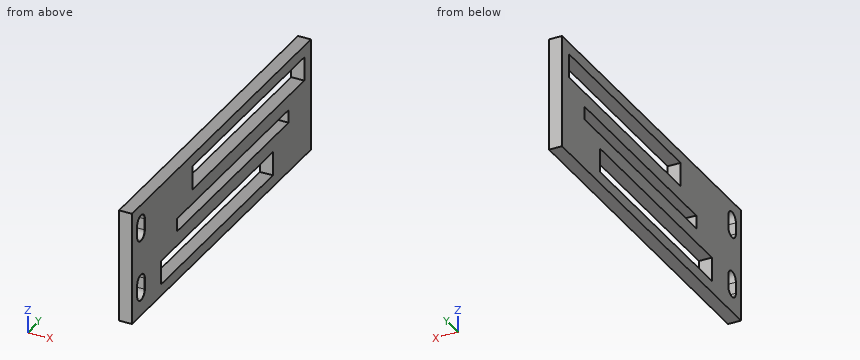
```python
from build123d import *

# Parameters (mm, degrees)
SKETCH1_W                = 26
SKETCH1_H                = 80
BOSS_EXTRUDE1_DEPTH      = 3
SKETCH2_W                = 5.5
SKETCH2_H                = 50
SKETCH2_W_2              = 3
CUT_EXTRUDE1_DEPTH       = 3
M3_START                 = -1
M3_CLEARANCE_SLOT1_DEPTH = 5


with BuildPart() as part:
    # Sketch1 → Boss-Extrude1 (new body)
    with BuildSketch(Plane(origin=(0, 0, 0), x_dir=(0, 0, -1), z_dir=(1, 0, 0))):
        with Locations((13, 40)):
            Rectangle(SKETCH1_W, SKETCH1_H)
    extrude(amount=BOSS_EXTRUDE1_DEPTH)

    # Sketch2 → Cut-Extrude1 (cut)
    with BuildSketch(Plane(origin=(3, 0, 0), x_dir=(0, 0, -1), z_dir=(1, 0, 0))):
        with Locations((5.425, 52)):
            Rectangle(SKETCH2_W, SKETCH2_H)
        with Locations((13, 45)):
            Rectangle(SKETCH2_W_2, SKETCH2_H)
        with Locations((20.575, 38)):
            Rectangle(SKETCH2_W, SKETCH2_H)
    extrude(amount=-CUT_EXTRUDE1_DEPTH, mode=Mode.SUBTRACT)

    # M3 Clearance Slot1: read off the stored shape, not the designer's step
    # M3 Clearance Slot1 outline → M3 Clearance Slot1 (cut)
    with BuildSketch(Plane.YZ.offset(M3_START)):
        with BuildLine():
            Line((5.7, -20.725), (5.7, -18.125))
            ThreePointArc((5.7, -18.125), (4, -16.425), (2.3, -18.125))
            Line((2.3, -18.125), (2.3, -20.725))
            ThreePointArc((2.3, -20.725), (4, -22.425), (5.7, -20.725))
        make_face()
        with BuildLine():
            ThreePointArc((5.7, -4.125), (4, -2.425), (2.3, -4.125))
            Line((2.3, -4.125), (2.3, -6.725))
            ThreePointArc((2.3, -6.725), (4, -8.425), (5.7, -6.725))
            Line((5.7, -6.725), (5.7, -4.125))
        make_face()
    extrude(amount=M3_CLEARANCE_SLOT1_DEPTH, mode=Mode.SUBTRACT)

    # M3 Clearance Slot1 2: loft between two sections, ruled curve by curve
    m3_clearance_slot1_2_from = [
        Edge.make_three_point_arc((2.975, 5.7, -18.125), (2.975, 5.202081528, -16.922918472), (2.975, 4, -16.425)),
        Edge.make_three_point_arc((2.975, 4, -16.425), (2.975, 2.797918472, -16.922918472), (2.975, 2.3, -18.125)),
        Edge.make_three_point_arc((2.975, 2.3, -20.725), (2.975, 2.797918472, -21.927081528), (2.975, 4, -22.425)),
        Edge.make_three_point_arc((2.975, 4, -22.425), (2.975, 5.202081528, -21.927081528), (2.975, 5.7, -20.725)),
        Edge.make_line((2.975, 2.3, -18.125), (2.975, 2.3, -20.725)),
        Edge.make_line((2.975, 5.7, -18.125), (2.975, 5.7, -20.725)),
    ]
    m3_clearance_slot1_2_to = [
        Edge.make_three_point_arc((3, 5.725, -18.125), (3, 5.219759198, -16.905240802), (3, 4, -16.4)),
        Edge.make_three_point_arc((3, 4, -16.4), (3, 2.780240802, -16.905240802), (3, 2.275, -18.125)),
        Edge.make_three_point_arc((3, 2.275, -20.725), (3, 2.780240802, -21.944759198), (3, 4, -22.45)),
        Edge.make_three_point_arc((3, 4, -22.45), (3, 5.219759198, -21.944759198), (3, 5.725, -20.725)),
        Edge.make_line((3, 2.275, -18.125), (3, 2.275, -20.725)),
        Edge.make_line((3, 5.725, -18.125), (3, 5.725, -20.725)),
    ]
    m3_clearance_slot1_2 = Solid(Shell([*[Face.make_surface_from_curves(m3_clearance_slot1_2_from[k], m3_clearance_slot1_2_to[k]) for k in range(6)], Face(Wire(m3_clearance_slot1_2_from)), Face(Wire(m3_clearance_slot1_2_to))]))
    add(m3_clearance_slot1_2, mode=Mode.SUBTRACT)

    # M3 Clearance Slot1 3: loft between two sections, ruled curve by curve
    m3_clearance_slot1_3_from = [
        Edge.make_three_point_arc((2.975, 5.7, -4.125), (2.975, 5.202081528, -2.922918472), (2.975, 4, -2.425)),
        Edge.make_three_point_arc((2.975, 4, -2.425), (2.975, 2.797918472, -2.922918472), (2.975, 2.3, -4.125)),
        Edge.make_three_point_arc((2.975, 2.3, -6.725), (2.975, 2.797918472, -7.927081528), (2.975, 4, -8.425)),
        Edge.make_three_point_arc((2.975, 4, -8.425), (2.975, 5.202081528, -7.927081528), (2.975, 5.7, -6.725)),
        Edge.make_line((2.975, 2.3, -4.125), (2.975, 2.3, -6.725)),
        Edge.make_line((2.975, 5.7, -4.125), (2.975, 5.7, -6.725)),
    ]
    m3_clearance_slot1_3_to = [
        Edge.make_three_point_arc((3, 5.725, -4.125), (3, 5.219759198, -2.905240802), (3, 4, -2.4)),
        Edge.make_three_point_arc((3, 4, -2.4), (3, 2.780240802, -2.905240802), (3, 2.275, -4.125)),
        Edge.make_three_point_arc((3, 2.275, -6.725), (3, 2.780240802, -7.944759198), (3, 4, -8.45)),
        Edge.make_three_point_arc((3, 4, -8.45), (3, 5.219759198, -7.944759198), (3, 5.725, -6.725)),
        Edge.make_line((3, 2.275, -4.125), (3, 2.275, -6.725)),
        Edge.make_line((3, 5.725, -4.125), (3, 5.725, -6.725)),
    ]
    m3_clearance_slot1_3 = Solid(Shell([*[Face.make_surface_from_curves(m3_clearance_slot1_3_from[k], m3_clearance_slot1_3_to[k]) for k in range(6)], Face(Wire(m3_clearance_slot1_3_from)), Face(Wire(m3_clearance_slot1_3_to))]))
    add(m3_clearance_slot1_3, mode=Mode.SUBTRACT)


solid = part.part
```
Could you check a few things on this model? Use its own coordinates, in mm. Give positions to 0.01 mm unless a question says otherwise; leave off trailing zeros. Order: outer loops, then holes, each group sorted by start corner. A loop starts at its lowest first (then second) coordinate and runs counter-clockwise, first axis right, second up.
Q1. Suppose I cut it at D-D, the plane y = 47. Write out the boundary of the cut face in (x, z) (3 decimals).
Q2. Suppose I cut it at C-C, the plane x = 1.65. Write out the boundary of the cut face in (y, z) (3 decimals), and give its area (3 significant figures).
Q3. I'm going to push a flat-ended pin straight in: P1, Ø1.5, axis at x = 2, y = 58.5, coming from the +Z side. Where does the tip first touch, or does it pass through?
Q4. Suppose I cut it at B-B, the plane y = 23.5. Write out the boundary of the cut face in (x, z) (3 decimals), and give its area (3 significant figures).
Q5. Suppose I cut it at A-A, the plane y = 14. Write out the boundary of the cut face in (x, z) (3 decimals).
Q6. If I drill on line 1 along Z through (x, y) = (2.1, 40.5) (3 decimals); line 2 along Y through (x, z) = (0.9, -4); line 3 along Y through (x, z) = (1.1, -19.25), over which ranges is the centre line in solid material (lowest first)?
Solution:
1. outline: (0, -26) - (3, -26) - (3, -23.325) - (0, -23.325) - close; (0, -17.825) - (3, -17.825) - (3, -14.5) - (0, -14.5) - close; (0, -11.5) - (3, -11.5) - (3, -8.175) - (0, -8.175) - close; (0, -2.675) - (3, -2.675) - (3, 0) - (0, 0) - close
2. outline: (0, -26) - (80, -26) - (80, 0) - (0, 0) - close; hole (2.3, -20.725) arc R1.7 ccw to (5.7, -20.725) - (5.7, -18.125) arc R1.7 ccw to (2.3, -18.125) - close; hole (2.3, -6.725) arc R1.7 ccw to (5.7, -6.725) - (5.7, -4.125) arc R1.7 ccw to (2.3, -4.125) - close; hole (13, -23.325) - (63, -23.325) - (63, -17.825) - (13, -17.825) - close; hole (20, -14.5) - (70, -14.5) - (70, -11.5) - (20, -11.5) - close; hole (27, -8.175) - (77, -8.175) - (77, -2.675) - (27, -2.675) - close
2. area: 1,340 mm2
3. P1: stops at z = 0
4. outline: (0, -26) - (3, -26) - (3, -23.325) - (0, -23.325) - close; (0, -17.825) - (3, -17.825) - (3, -14.5) - (0, -14.5) - close; (0, -11.5) - (3, -11.5) - (3, 0) - (0, 0) - close
4. area: 52.5 mm2
5. outline: (0, -26) - (3, -26) - (3, -23.325) - (0, -23.325) - close; (0, -17.825) - (3, -17.825) - (3, 0) - (0, 0) - close
6. line 1: z = -26 to -23.325, -17.825 to -14.5, -11.5 to -8.175, -2.675 to 0
6. line 2: y = 0 to 2.3, 5.7 to 27, 77 to 80
6. line 3: y = 0 to 2.3, 5.7 to 13, 63 to 80
